The listing builds one solid part. Answer for the finished solid, in the listing's coordinates (mm). A direction names the side the tool comes from. Round coordinates to 2 decimals unless told otherwise and drop trailing zeros. Order: outer loops, then holes, each group sorted by start corner. A loop starts at its lowest first (then second) coordinate and runs counter-clockwise, first axis right, second up. Notation, with made-up numbers: (0.5, 31.5) - (22.5, 31.5) arc R23 cw to (22.5, 48.5) - close; hole circle Ø7 at (-10.75, 18). An arc over 180 degrees is marked (long way). Write item = value, one per line.
from build123d import *

# Parameters (mm, degrees)
F0_R     = 12.7
F1_DEPTH = 25.4
F3_DEPTH = 25.4
F4_R     = 12.7


with BuildPart() as f1:
    # F0 (on Front) → F1 (new body)
    with BuildSketch(Plane.XZ):
        with BuildLine():
            Line((60.995375, -7.947213), (-26.366752, 51.187115))
            ThreePointArc((-26.366752, 51.187115), (-52.510884, 52.589386), (-66.004625, 30.152787))
            Line((-66.004625, 30.152787), (-66.004625, -20.647213))
            Line((-66.004625, -20.647213), (60.995375, -20.647213))
            Line((60.995375, -20.647213), (60.995375, -7.947213))
        make_face()
        with Locations((-40.604625, 30.152787)):
            Circle(F0_R, mode=Mode.SUBTRACT)
    extrude(amount=F1_DEPTH)

    # F2 (on face) → F3 (join)
    with BuildSketch(Plane.XZ.offset(25.4)):
        with BuildLine():
            Line((60.746003, -20.647213), (60.746003, -9.422782))
            Line((60.746003, -9.422782), (-15.164001, -9.422782))
            Line((-15.164001, -9.422782), (-15.164001, 30.397678))
            ThreePointArc((-15.164001, 30.397678), (-17.383882, 40.782384), (-23.655506, 49.351907))
            Line((-23.655506, 49.351907), (-26.366752, 51.187115))
            ThreePointArc((-26.366752, 51.187115), (-50.57153, 53.515595), (-65.641578, 34.431919))
            ThreePointArc((-65.641578, 34.431919), (-65.9137, 32.300039), (-66.004625, 30.152787))
            Line((-66.004625, 30.152787), (-66.004625, -20.647213))
            Line((-66.004625, -20.647213), (-65.891497, -20.647213))
            Line((-65.891497, -20.647213), (60.746003, -20.647213))
        make_face()
        with BuildLine():
            ThreePointArc((-53.112497, 32.353501), (-39.583159, 43.059745), (-27.864001, 30.397678))
            ThreePointArc((-27.864001, 30.397678), (-27.912124, 29.293135), (-28.056129, 28.196964))
            ThreePointArc((-28.056129, 28.196964), (-42.682993, 17.624005), (-53.112497, 32.353501))
        make_face(mode=Mode.SUBTRACT)
    extrude(amount=F3_DEPTH)

    # F4
    f4_edges = [f1.edges().sort_by_distance(p)[0] for p in [
        (60.746003, -50.8, -15.034997),
    ]]
    fillet(f4_edges, radius=F4_R)


solid = f1.part
Q1. Section C-C on x = -46 is taken. Determine the outline of the cut face in (y, z).
Model answer:
outline = (-50.8, -20.65) - (0, -20.65) - (0, 18.66) - (-50.8, 18.66) - close; (-50.8, 41.88) - (-25.4, 41.88) - (-25.4, 41.65) - (0, 41.65) - (0, 54.97) - (-50.8, 54.97) - close
Q2. Section A-A on y = -35 is taken. Determine the outline of the cut face in (x, z).
Model answer:
outline = (-66, -20.65) - (60.75, -20.65) - (60.75, -9.42) - (-15.16, -9.42) - (-15.16, 30.4) arc R25.4 ccw to (-23.66, 49.35) - (-26.37, 51.19) arc R25.4 ccw to (-65.64, 34.43) arc R25.4 ccw to (-66, 30.15) - close; hole (-53.11, 32.35) arc R12.7 ccw (long way) to (-28.06, 28.2) arc R12.7 ccw to (-27.86, 30.4) arc R12.7 ccw to start
Q3. Section B-B on z = 19 is taken. Determine the outline of the cut face in (x, y).
Model answer:
outline = (-66, -50.8) - (-46.68, -50.8) - (-46.68, 0) - (-66, 0) - close; (-34.53, -50.8) - (-15.16, -50.8) - (-15.16, -25.4) - (21.18, -25.4) - (21.18, 0) - (-34.53, 0) - close
Q4. Find the intervals of material crossed by line 1 (Y direction, x = -11.5, z = 11); line 2 (Z direction, x = 44, y = -33.5); line 3 (X direction, y = -32, z = 3), in increasing order. Write a range as from..to.
Model answer:
line_1 = -25.4..0
line_2 = -20.65..-9.42
line_3 = -66..-15.16
Q5. Determine the mould class of faces 4 (the face through (-3, -25, -20.647)), 5 (the face through (60.995, -13, -14)), 6 (the face through (-39.848, -37.922, 43.077)) for opening direction Z: released by +Z, released by -Z, zero draft, split by the parting line, or undercut.
Model answer:
face_4 = released by -Z
face_5 = zero draft
face_6 = undercut
Q6. For faces 1 (the face through (60.746, -32, -15)), 2 (the face through (-35, -50.8, 10)), 3 (the face through (-15.164, -38, 10)), determine the directions among +Z, -Z, +X, -X, +Y, -Y from which every point of the face is accessible in a straight line to the end or side of a thin tool.
Model answer:
face_1 = +Z, -Z, +X, -Y
face_2 = +Z, -Z, +X, -X, -Y
face_3 = +Z, +X, -Y
Q7. Flat-ended cylindrical pins translate along their axes: P1, Ø2, axis at x = -15, z = 41.5, coming from the +Y side; P2, Ø12, axis at x = 13.5, y = -40.5, coming from the +Z side; P3, Ø12, axis at x = 19, y = -22, coming from the +Z side; P4, Ø3.5, axis at y = -33, z = -17, coming from the +X side. Find the tip coordinate at first contact, or state that the pin passes through.
Model answer:
P1 = 0
P2 = -9.42
P3 = 24.54
P4 = 60.75
Q8. Section D-D on z = 46 is taken. Determine the outline of the cut face in (x, y), then the cut area to 3 significant figures.
Model answer:
outline = (-60.45, -50.8) - (-20.52, -50.8) - (-20.52, -25.4) - (-18.7, -25.4) - (-18.7, 0) - (-60.45, 0) - close
area = 2,070 mm^2
